Could you check a few things on this model? Use its own coordinates, in mm. A direction names the side the tool comes from. Round coordinates to 2 decimals unless told otherwise and drop trailing zeros. Order: outer loops, then holes, each group sorted by start corner. A loop starts at its lowest first (then second) coordinate and runs counter-clockwise, first axis right, second up. Notation, with made-up numbers: (-0.75, 54) - (3.25, 54) arc R37 cw to (3.25, 90) - close; hole circle Ø2 at (-34, 10.5). An arc over 180 degrees is marked (long way). Use one line per item in the form item = value.
from build123d import *

# Parameters (mm, degrees)
BOSS_EXTRUDE1_DEPTH     = 110
BOSS_EXTRUDE2_REACH     = 144.215
SKETCH2_W               = 7
SKETCH2_H               = 20
SKETCH4_W               = 7
SKETCH4_H               = 20
BOSS_EXTRUDE3_DEPTH     = 14.5
CUT_EXTRUDE1_DEPTH      = 145.066443005
CUT_EXTRUDE1_DEPTH_BACK = 145.066443005
SKETCH5_R               = 2


with BuildPart() as part:
    # Sketch1 → Boss-Extrude1 (new body)
    with BuildSketch(Plane.XY):
        Polygon((0, 0), (0, -17.14826885), (12.85173115, -30), (72.14826885, -30), (85, -17.14826885), (85, 0), (81, 0), (81, -15.4914146), (70.4914146, -26), (14.5085854, -26), (4, -15.4914146), (4, 0), align=None)
    extrude(amount=BOSS_EXTRUDE1_DEPTH)

    # Sketch2 → Boss-Extrude2 (add, up to next)
    with BuildSketch(Plane.XZ.offset(30), mode=Mode.PRIVATE) as boss_extrude2_sk1:
        with Locations((6.8, 25)):
            Rectangle(SKETCH2_W, SKETCH2_H)
    boss_extrude2_tool1 = extrude(boss_extrude2_sk1.sketch, amount=-BOSS_EXTRUDE2_REACH, mode=Mode.PRIVATE) - part.part
    # Sketch2 → Boss-Extrude2 (add, up to next)
    with BuildSketch(Plane.XZ.offset(30), mode=Mode.PRIVATE) as boss_extrude2_sk2:
        with Locations((79.2, 85)):
            Rectangle(SKETCH2_W, SKETCH2_H)
    boss_extrude2_tool2 = extrude(boss_extrude2_sk2.sketch, amount=-BOSS_EXTRUDE2_REACH, mode=Mode.PRIVATE) - part.part
    add(boss_extrude2_tool1.solids().sort_by_distance((6.8, -30, 25))[0])
    add(boss_extrude2_tool2.solids().sort_by_distance((79.2, -30, 85))[0])

    # Sketch4 → Boss-Extrude3 (add)
    with BuildSketch(Plane.XZ.offset(30)):
        with Locations((6.8, 25)):
            Rectangle(SKETCH4_W, SKETCH4_H)
        with Locations((79.2, 85)):
            Rectangle(SKETCH4_W, SKETCH4_H)
    extrude(amount=BOSS_EXTRUDE3_DEPTH)

    # Sketch5 → Cut-Extrude1 (cut, two sides: drawn at the far end of the back side and taken through both)
    with BuildSketch(Plane.ZY.offset(-3.3).offset(-CUT_EXTRUDE1_DEPTH_BACK)):
        with Locations((20, -38.15)):
            Circle(SKETCH5_R)
        with Locations((30, -38.15)):
            Circle(SKETCH5_R)
        with Locations((80, -38.15)):
            Circle(SKETCH5_R)
        with Locations((90, -38.15)):
            Circle(SKETCH5_R)
    extrude(amount=CUT_EXTRUDE1_DEPTH + CUT_EXTRUDE1_DEPTH_BACK, mode=Mode.SUBTRACT)


solid = part.part
Item 1: Imagine slicing it at A-A on z = 80. Please give me the cut outline in (x, y), plus the area to 3 significant figures.
Found:
outline = (0, -17.15) - (12.85, -30) - (72.15, -30) - (75.7, -26.45) - (75.7, -36.15) - (82.7, -36.15) - (82.7, -19.45) - (85, -17.15) - (85, 0) - (81, 0) - (81, -15.49) - (70.49, -26) - (14.51, -26) - (4, -15.49) - (4, 0) - (0, 0) - close; (75.7, -44.5) - (82.7, -44.5) - (82.7, -40.15) - (75.7, -40.15) - close
area = 616 mm2
Item 2: Imagine slicing it at D-D on y = -22.5. Please give me the cut outline in (x, z).
Found:
outline = (3.3, 15) - (5.35, 15) - (5.35, 0) - (11.01, 0) - (11.01, 110) - (5.35, 110) - (5.35, 35) - (3.3, 35) - close; (73.99, 0) - (79.65, 0) - (79.65, 75) - (82.7, 75) - (82.7, 95) - (79.65, 95) - (79.65, 110) - (73.99, 110) - close
Item 3: For faces 4 (the face through (9.33, -20.82, 54.23)), 5 (the face through (42, -30, 54)), 6 (the face through (7, -35, 15)), 7 (the face through (7, -35, 35)), which set-ups out of +Z, -Z, +X, -X, +Y, -Y let a thin tool reach every point of the face, with its end or its side?
Found:
face_4 = +Z, -Z, +Y
face_5 = +Z, -Z, -Y
face_6 = -Z, -X, -Y
face_7 = +Z, -X, -Y
Item 4: Imagine slicing it at C-C on z = 30. Please give me the cut outline in (x, y).
Found:
outline = (0, -17.15) - (3.3, -20.45) - (3.3, -36.15) - (10.3, -36.15) - (10.3, -27.45) - (12.85, -30) - (72.15, -30) - (85, -17.15) - (85, 0) - (81, 0) - (81, -15.49) - (70.49, -26) - (14.51, -26) - (4, -15.49) - (4, 0) - (0, 0) - close; (3.3, -44.5) - (10.3, -44.5) - (10.3, -40.15) - (3.3, -40.15) - close
Item 5: I need wall thicknesses on L1, parallel to Z at x = 7, y = -38.15; L2, parallel to Z at x = 81, y = -38; L3, parallel to X at y = -9, z = 29. Which ranges of each line are inside material? Lowest first, please.
Found:
L1 = 15 to 18, 22 to 28, 32 to 35
L2 = 75 to 78.01, 81.99 to 88.01, 91.99 to 95
L3 = 0 to 4, 81 to 85
Item 6: Will these pins go through, and if not, where does the flat tip stop? P1, Ø17, axis at x = 38.5, z = 28.5, coming from the +Y side; P2, Ø4.5, axis at y = -38.15, z = 20, coming from the +X side; P3, Ø6, axis at x = 68.5, z = 35.5, coming from the -Y side.
Found:
P1 = -26
P2 = 10.3
P3 = -30
Item 7: Imagine slicing it at B-B on y = -38.15. Please give me the cut outline in (x, z), plus the area to 3 significant figures.
Found:
outline = (3.3, 15) - (10.3, 15) - (10.3, 18) - (3.3, 18) - close; (3.3, 22) - (10.3, 22) - (10.3, 28) - (3.3, 28) - close; (3.3, 32) - (10.3, 32) - (10.3, 35) - (3.3, 35) - close; (75.7, 75) - (82.7, 75) - (82.7, 78) - (75.7, 78) - close; (75.7, 82) - (82.7, 82) - (82.7, 88) - (75.7, 88) - close; (75.7, 92) - (82.7, 92) - (82.7, 95) - (75.7, 95) - close
area = 168 mm2
Item 8: If we mould it in two halves opening along X, with no side actions, what happens to faces 1 (the face through (39, -27, 110)), 2 (the face through (82.7, -32, 85)), 3 (the face through (43, -26, 54))? For each: released by +X, released by -X, zero draft, split by the parting line, or undercut.
Found:
face_1 = zero draft
face_2 = released by +X
face_3 = undercut
